Job drawing, mm, ordinate dimensions from the low corner. One solid piece. Give positions to 0.01 mm unless a question says otherwise; leave off trailing zeros. Loops run counter-clockwise (first coordinate to the right, second up) from the corner with the lowest first, then second, coordinate; pieces in that order, holes last. Notation, with made-up numbers: M 28.5,-2.75 L 79.5,-2.75 A30 ccw 79.5,19.25 Z; hole C 49.5,-25.75 d7. An arc over 180 degrees is marked long. Answer in a Markdown table with one row per item.
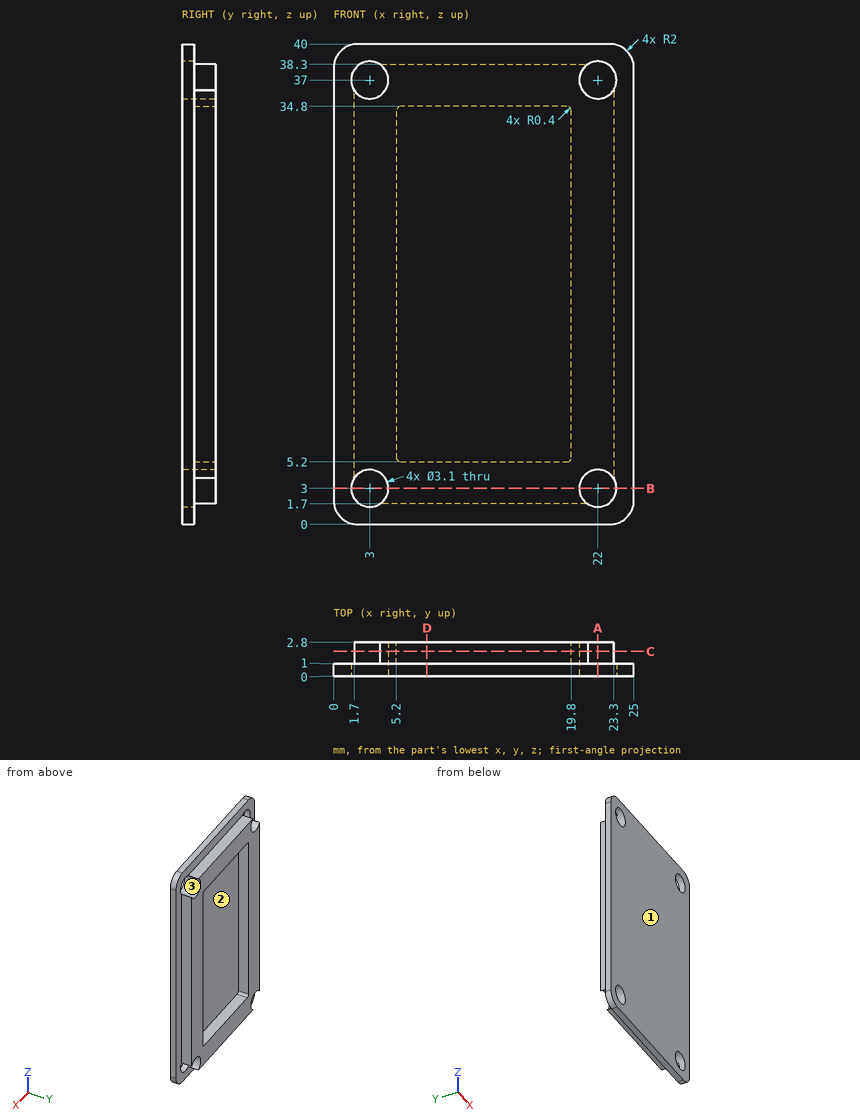
(1) Saw through at B-B (z = 3). Write the cut outline in (x, y), plus the area to 3 significant figures.
Recorded:
| item | result |
|---|---|
| outline | M 0,0 L 1.45,0 L 1.45,1 L 0,1 Z; M 4.55,0 L 20.45,0 L 20.45,2.8 L 4.55,2.8 Z; M 23.55,0 L 25,0 L 25,1 L 23.55,1 Z |
| area | 47.4 mm^2 |
(2) Pull direction Z, two halves, no side cores. Call the marked faces 1, 2 and 3: +Z half, -Z half, draft (parallel to the pull), parting line (faces both ways), or undercut.
Recorded:
| item | result |
|---|---|
| face 1 | draft |
| face 2 | undercut |
| face 3 | undercut |
(3) Pin check, flat tips, straight feed: pin 1 Ø0.9 at (x, y) = (8.5, 2) entering from +Z; pin 2 Ø7.5 at (x, z) = (12.5, 14.5) entering from +Y; pin 3 Ø0.5 at (y, z) = (2, 24.5) entering from +X. Stop position of each tip, or through.
Recorded:
| item | result |
|---|---|
| pin 1 | stops at z = 38.3 |
| pin 2 | stops at y = 1 |
| pin 3 | stops at x = 23.3 |
(4) Saw through at D-D (x = 7.75). Write the cut outline in (y, z).
Recorded:
| item | result |
|---|---|
| outline | M 0,0 L 1,0 L 1,1.7 L 2.8,1.7 L 2.8,5.2 L 1,5.2 L 1,34.8 L 2.8,34.8 L 2.8,38.3 L 1,38.3 L 1,40 L 0,40 Z |
(5) Saw through at A-A (x = 22). Write the cut outline in (y, z), plus the area to 3 significant figures.
Recorded:
| item | result |
|---|---|
| outline | M 0,0 L 1,0 L 1,1.45 L 0,1.45 Z; M 0,4.55 L 2.8,4.55 L 2.8,35.45 L 0,35.45 Z; M 0,38.55 L 1,38.55 L 1,40 L 0,40 Z |
| area | 89.4 mm^2 |
(6) Saw through at C-C (y = 2.05). Write the cut outline in (x, z).
Recorded:
| item | result |
|---|---|
| outline | M 1.7,3.84 A1.55 cw long 3.84,1.7 L 21.16,1.7 A1.55 cw long 23.3,3.84 L 23.3,36.16 A1.55 cw long 21.16,38.3 L 3.84,38.3 A1.55 cw long 1.7,36.16 Z; hole M 5.2,5.6 A0.4 ccw 5.6,5.2 L 19.4,5.2 A0.4 ccw 19.8,5.6 L 19.8,34.4 A0.4 ccw 19.4,34.8 L 5.6,34.8 A0.4 ccw 5.2,34.4 Z |
(7) Drill centre lines: line 1 along X through (y, z) = (0.95, 38); line 2 along Z through (x, y) = (5.75, 1.45); line 3 along Z through (x, y) = (3, 1.7). Where is each one in solid material? Low to high.
Recorded:
| item | result |
|---|---|
| line 1 | x = 0 to 1.82, 4.18 to 20.82, 23.18 to 25 |
| line 2 | z = 1.7 to 5.2, 34.8 to 38.3 |
| line 3 | z = 4.55 to 35.45 |
